Can you work these out from the model? Positions are in its coordinate system, mm. A direction names the side the tool comes from. Give positions to 0.01 mm unless a question says otherwise; leave off trailing zeros. Loops run counter-clockwise (first coordinate to the right, second up) from the corner with the lowest first, then second, coordinate; pieces in that order, holes last. Notation, with made-up numbers: M 15,-25.5 L 67,-25.5 A6 ccw 67,-21.5 Z; hole C 41.5,62 d3. An arc over 180 degrees is marked long. Use CSV: the item, a comma, the result in double quotes.
from build123d import *

# Parameters (mm, degrees)
SKETCH1_W           = 21
SKETCH1_H           = 40
BOSS_EXTRUDE1_DEPTH = 12
CUT_EXTRUDE1_REACH  = 48.744
SKETCH2_R           = 6
CUT_EXTRUDE2_REACH  = 48.744
SKETCH3_R           = 2
SKETCH4_R           = 3.75
CUT_EXTRUDE3_DEPTH  = 1.5
FILLET1_R           = 2


with BuildPart() as part:
    # Sketch1 → Boss-Extrude1 (new body)
    with BuildSketch(Plane.XY):
        with Locations((10.5, 20)):
            Rectangle(SKETCH1_W, SKETCH1_H)
    extrude(amount=BOSS_EXTRUDE1_DEPTH)

    # Sketch2 → Cut-Extrude1 (cut, up to next)
    with BuildSketch(Plane.XY.offset(12), mode=Mode.PRIVATE) as cut_extrude1_sk1:
        with Locations((12.5, 20)):
            Circle(SKETCH2_R)
    cut_extrude1_tool1 = extrude(cut_extrude1_sk1.sketch, amount=-CUT_EXTRUDE1_REACH, mode=Mode.PRIVATE) & part.part
    add(cut_extrude1_tool1.solids().sort_by_distance((12.5, 20, 12))[0], mode=Mode.SUBTRACT)

    # Sketch3 → Cut-Extrude2 (cut, up to next)
    with BuildSketch(Plane.ZY, mode=Mode.PRIVATE) as cut_extrude2_sk1:
        with Locations((6, 30)):
            Circle(SKETCH3_R)
    cut_extrude2_tool1 = extrude(cut_extrude2_sk1.sketch, amount=-CUT_EXTRUDE2_REACH, mode=Mode.PRIVATE) & part.part
    # Sketch3 → Cut-Extrude2 (cut, up to next)
    with BuildSketch(Plane.ZY, mode=Mode.PRIVATE) as cut_extrude2_sk2:
        with Locations((6, 10)):
            Circle(SKETCH3_R)
    cut_extrude2_tool2 = extrude(cut_extrude2_sk2.sketch, amount=-CUT_EXTRUDE2_REACH, mode=Mode.PRIVATE) & part.part
    add(cut_extrude2_tool1.solids().sort_by_distance((0, 30, 6))[0], mode=Mode.SUBTRACT)
    add(cut_extrude2_tool2.solids().sort_by_distance((0, 10, 6))[0], mode=Mode.SUBTRACT)

    # Sketch4 → Cut-Extrude3 (cut)
    with BuildSketch(Plane.ZY):
        with Locations((6, 30)):
            Circle(SKETCH4_R)
        with Locations((6, 10)):
            Circle(SKETCH4_R)
    extrude(amount=-CUT_EXTRUDE3_DEPTH, mode=Mode.SUBTRACT)

    # Fillet1
    fillet1_edges = [part.edges().sort_by_distance(p)[0] for p in [
        (0, 40, 6),
        (21, 40, 6),
        (21, 0, 6),
        (0, 0, 6),
    ]]
    fillet(fillet1_edges, radius=FILLET1_R)


solid = part.part
Q1. I'm going to push a flat-ended pin straight in: P1, Ø1, axis at y = 12, z = 6, coming from the -X side. Where does the tip first touch, or does it pass through?
Model answer:
P1,"x = 1.5"
Q2. I want a section at A-A, the plane z = 6. Please give me the cut outline in (x, y).
Model answer:
outline,"M 0,2 A2 ccw 2,0 L 19,0 A2 ccw 21,2 L 21,8 L 1.5,8 L 1.5,6.25 L 0,6.25 Z; M 0,13.75 L 1.5,13.75 L 1.5,12 L 21,12 L 21,28 L 1.5,28 L 1.5,26.25 L 0,26.25 Z; M 0,33.75 L 1.5,33.75 L 1.5,32 L 21,32 L 21,38 A2 ccw 19,40 L 2,40 A2 ccw 0,38 Z; hole C 12.5,20 d12"
Q3. If we mould it in two halves opening along Z, with no side actions, what happens to faces 1 (the flat face through (6, 20, 0)), 2 (the flat face through (10, 0, 6)), 3 (the cylindrical face through (0.74, 33.718, 5.512))? For each: released by +Z, released by -Z, zero draft, split by the parting line, or undercut.
Model answer:
face 1,"released by -Z"
face 2,"zero draft"
face 3,"undercut"
Q4. Please list where these lines run through material, in increasing order: L1, parallel to Y at x = 3.25, z = 6.75; L2, parallel to Y at x = 13.25, z = 6.5; L3, parallel to Y at x = 10.5, z = 6. Write a range as from..to.
Model answer:
L1,"0..8.15, 11.85..28.15, 31.85..40"
L2,"0..8.06, 11.94..14.05, 25.95..28.06, 31.94..40"
L3,"0..8, 12..14.34, 25.66..28, 32..40"
Q5. I want a section at B-B, the plane x = 17.25. Please give me the cut outline in (y, z).
Model answer:
outline,"M 0,0 L 16.33,0 L 16.33,12 L 0,12 Z; M 23.67,0 L 40,0 L 40,12 L 23.67,12 Z; hole C 10,6 d4; hole C 30,6 d4"
Q6. I want a section at C-C, the plane y = 10. Please give me the cut outline in (x, z).
Model answer:
outline,"M 0,0 L 21,0 L 21,4 L 1.5,4 L 1.5,2.25 L 0,2.25 Z; M 0,9.75 L 1.5,9.75 L 1.5,8 L 21,8 L 21,12 L 0,12 Z"
Q7. For faces 4 (the flat face through (21, 20, 6)), 5 (the flat face through (1.5, 28, 8)), which set-ups out of +Z, -Z, +X, -X, +Y, -Y let a thin tool reach every point of the face, with its end or its side?
Model answer:
face 4,"+Z, -Z, +X, +Y, -Y"
face 5,"-X"
Q8. I want a section at D-D, the plane x = 12.5. Please give me the cut outline in (y, z), then the cut area to 3 significant figures.
Model answer:
outline,"M 0,0 L 14,0 L 14,12 L 0,12 Z; M 26,0 L 40,0 L 40,12 L 26,12 Z; hole C 10,6 d4; hole C 30,6 d4"
area,"311 mm2"
